Geometry: final body of the model. Coordinates: model frame, mm. Give positions to 0.01 mm unless a question says otherwise; leave off trailing zeros. Loops run counter-clockwise (first coordinate to the right, second up) from the corner with the lowest first, then second, coordinate; pieces in that order, holes last.
```python
from build123d import *

# Parameters (mm, degrees)
BOSS_EXTRUDE1_DEPTH = 6.35
CUT_EXTRUDE1_DEPTH  = 6.35
CUT_EXTRUDE2_DEPTH  = 6.35
MODEL_7_R           = 1.7
MODEL_7_R_2         = 1.5
MODEL_7_R_3         = 2.25
MODEL_7_R_4         = 1.6
MODEL_7_R_5         = 2
CUT_EXTRUDE3_DEPTH  = 6.35
MODEL_8_W           = 17.2
MODEL_8_H           = 5
CUT_EXTRUDE4_DEPTH  = 6.35


with BuildPart() as part:
    # Model → Boss-Extrude1 (new body)
    with BuildSketch(Plane.XY):
        Polygon((110, -105), (110, -100), (100, -90), (100, -74), (110, -64), (110, -36), (100, -26), (100, -20), (110, -10), (110, 10), (100, 20), (100, 26), (110, 36), (110, 64), (100, 74), (100, 90), (110, 100), (110, 105), (105, 110), (100, 110), (90, 100), (20, 100), (10, 110), (-10, 110), (-20, 100), (-90, 100), (-100, 110), (-105, 110), (-110, 105), (-110, 100), (-100, 90), (-100, 20), (-110, 10), (-110, -10), (-100, -20), (-100, -90), (-110, -100), (-110, -105), (-105, -110), (-100, -110), (-90, -100), (-20, -100), (-10, -110), (10, -110), (20, -100), (90, -100), (100, -110), (105, -110), align=None)
    extrude(amount=BOSS_EXTRUDE1_DEPTH)

    # Model<4> → Cut-Extrude1 (cut)
    with BuildSketch(Plane.XY):
        Polygon((-47.489728574, 85), (-57.489728574, 75), (-57.489728574, 45), (-47.489728574, 35), (47.489728574, 35), (57.489728574, 45), (57.489728574, 75), (47.489728574, 85), align=None)
    extrude(amount=CUT_EXTRUDE1_DEPTH, mode=Mode.SUBTRACT)

    # Model<5> → Cut-Extrude2 (cut)
    with BuildSketch(Plane.XY):
        Polygon((57.489728574, -45), (47.489728574, -35), (-47.489728574, -35), (-57.489728574, -45), (-57.489728574, -75), (-47.489728574, -85), (47.489728574, -85), (57.489728574, -75), align=None)
    extrude(amount=CUT_EXTRUDE2_DEPTH, mode=Mode.SUBTRACT)

    # Model<7> → Cut-Extrude3 (cut)
    with BuildSketch(Plane.XY):
        with Locations((0, -104.75)):
            Circle(MODEL_7_R)
        with Locations((104.75, 0)):
            Circle(MODEL_7_R)
        with Locations((104.5, 104.5)):
            Circle(MODEL_7_R)
        with Locations((104.5, -104.5)):
            Circle(MODEL_7_R)
        with Locations((-95, 0)):
            Circle(MODEL_7_R_2)
        with Locations((-75, 0)):
            Circle(MODEL_7_R_2)
        with Locations((-73, 9)):
            Circle(MODEL_7_R_3)
        with Locations((-73, -9)):
            Circle(MODEL_7_R_3)
        with Locations((-97, -9)):
            Circle(MODEL_7_R_3)
        with Locations((-97, 9)):
            Circle(MODEL_7_R_3)
        with Locations((75, 50)):
            Circle(MODEL_7_R_2)
        with Locations((95, 50)):
            Circle(MODEL_7_R_2)
        with Locations((75, -50)):
            Circle(MODEL_7_R_2)
        with Locations((95, -50)):
            Circle(MODEL_7_R_2)
        with Locations((97, 59)):
            Circle(MODEL_7_R_3)
        with Locations((97, 41)):
            Circle(MODEL_7_R_3)
        with Locations((73, 41)):
            Circle(MODEL_7_R_3)
        with Locations((73, 59)):
            Circle(MODEL_7_R_3)
        with Locations((97, -41)):
            Circle(MODEL_7_R_3)
        with Locations((97, -59)):
            Circle(MODEL_7_R_3)
        with Locations((73, -59)):
            Circle(MODEL_7_R_3)
        with Locations((73, -41)):
            Circle(MODEL_7_R_3)
        with Locations((-104.75, 0)):
            Circle(MODEL_7_R)
        with Locations((0, 104.75)):
            Circle(MODEL_7_R)
        with Locations((-104.5, 104.5)):
            Circle(MODEL_7_R)
        with Locations((-104.5, -104.5)):
            Circle(MODEL_7_R)
        with Locations((-7, 30)):
            Circle(MODEL_7_R_4)
        with Locations((7, 30)):
            Circle(MODEL_7_R_4)
        with Locations((-7, -30)):
            Circle(MODEL_7_R_4)
        with Locations((7, -30)):
            Circle(MODEL_7_R_4)
        with Locations((70, -28)):
            Circle(MODEL_7_R_5)
        with Locations((-70, -28)):
            Circle(MODEL_7_R_5)
        with Locations((-70, 85)):
            Circle(MODEL_7_R_2)
        with Locations((-70, 75)):
            Circle(MODEL_7_R_2)
        with Locations((70, 85)):
            Circle(MODEL_7_R_2)
        with Locations((70, 75)):
            Circle(MODEL_7_R_2)
    extrude(amount=CUT_EXTRUDE3_DEPTH, mode=Mode.SUBTRACT)

    # Model<8> → Cut-Extrude4 (cut)
    with BuildSketch(Plane.XY):
        with BuildLine():
            Line((-81, -10.5), (-81, 10.5))
            ThreePointArc((-81, 10.5), (-85, 14.5), (-89, 10.5))
            Line((-89, 10.5), (-89, -10.5))
            ThreePointArc((-89, -10.5), (-85, -14.5), (-81, -10.5))
        make_face()
        with BuildLine():
            Line((89, 39.5), (89, 60.5))
            ThreePointArc((89, 60.5), (85, 64.5), (81, 60.5))
            Line((81, 60.5), (81, 39.5))
            ThreePointArc((81, 39.5), (85, 35.5), (89, 39.5))
        make_face()
        with BuildLine():
            Line((89, -60.5), (89, -39.5))
            ThreePointArc((89, -39.5), (85, -35.5), (81, -39.5))
            Line((81, -39.5), (81, -60.5))
            ThreePointArc((81, -60.5), (85, -64.5), (89, -60.5))
        make_face()
        with Locations((0, 19.5)):
            Rectangle(MODEL_8_W, MODEL_8_H)
        with Locations((0, -19.5)):
            Rectangle(MODEL_8_W, MODEL_8_H)
    extrude(amount=CUT_EXTRUDE4_DEPTH, mode=Mode.SUBTRACT)


solid = part.part
```
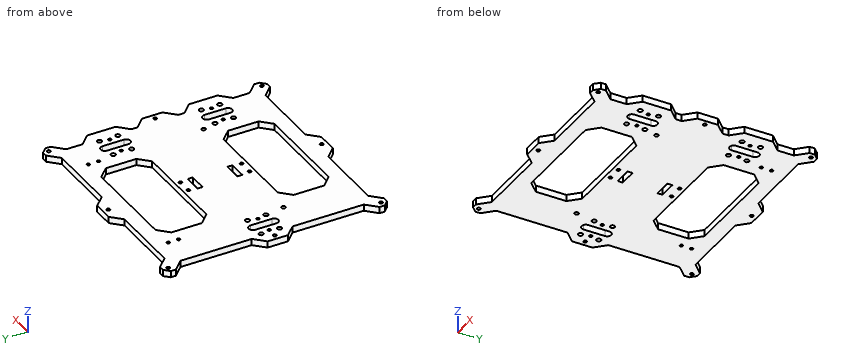
Q1. Section query A-A, the plane x = -30. Return loops of the section in (y, z), and give its area (3 significant figures).
Q2. Section query C-C, the plane x = 63.5. Return loops of the section in (y, z), and give its area (3 significant figures).
Q3. Material intervals for probe 1 along Y at (x, z) = (-21.5, 5); probe 2 along X at (y, z) = (-9.5, 0.5); probe 3 along Y at (x, z) = (-70, 3), sorted ascending.
Q4. Pin query (flat end, axial travel): pin 1 Ø1 at (y, z) = (-27, 5) entering from +X; pin 2 Ø1.9 at (y, z) = (67.5, 3) entering from +X; pin 3 Ø3 at (y, z) = (54.5, 2) entering from -X. Return the tip coordinate at first contact, or that it passes through.
Q5. Section query B-B, the plane z = 2.5. State how many separate pieces and enclosed holes the cut face has, and give its area (3 significant figures).
Resolved:
1. outline: (-100, 0) - (-85, 0) - (-85, 6.35) - (-100, 6.35) - close; (-35, 0) - (35, 0) - (35, 6.35) - (-35, 6.35) - close; (85, 0) - (100, 0) - (100, 6.35) - (85, 6.35) - close
1. area: 635 mm2
2. outline: (-100, 0) - (100, 0) - (100, 6.35) - (-100, 6.35) - close
2. area: 1,270 mm2
3. probe 1: y = -100 to -85, -35 to 35, 85 to 100
3. probe 2: x = -110 to -99.19, -94.81 to -89, -81 to -75.19, -70.81 to 110
3. probe 3: y = -100 to -30, -26 to 73.5, 76.5 to 83.5, 86.5 to 100
4. pin 1: stops at x = 101.5
4. pin 2: stops at x = 107.45
4. pin 3: stops at x = -100
5. separate pieces: 1
5. enclosed holes: 43
5. area: 30,400 mm2
